Drawing for the job (mm, zero at the part's lowest x, y, z). Round coordinates to 2 decimals unless told otherwise and drop trailing zeros. Write each loop counter-clockwise with the first axis right and the second up, starting at its lowest first coordinate (ties: lowest second). Pieces come first, ordered by that corner, then holes.
Item 1: Drop flat-ended pins along their axis: pin 1 Ø15 at (y, z) = (586, 457) entering from -X; pin 2 Ø12 at (x, y) = (802, 277) entering from -Z. Give the stop position or say it passes through.
Item 2: Mould opens along X. For the marked faces 1 and 2 say: +X half, -X half, draft (parallel to the pull), parting line (faces both ways), or undercut.
Item 3: Wall check: probe 1 along X at (y, z) = (46.5, 217); probe 2 along Z at (x, y) = (641, 485). Give the ranges that are in metal, low to high.
Item 4: Band-saw the part on D-D, the plane x = 477.5. Write the cut outline in (y, z), then the cut area to 3 significant figures.
Item 5: Band-saw the part on B-B, the plane y = 532. Write the cut outline in (x, z).
Item 6: Band-saw the part on C-C, the plane y = 336. Write the cut outline in (x, z).
Item 7: Band-saw the part on A-A, the plane z = 806.5. Write the cut outline in (x, y).
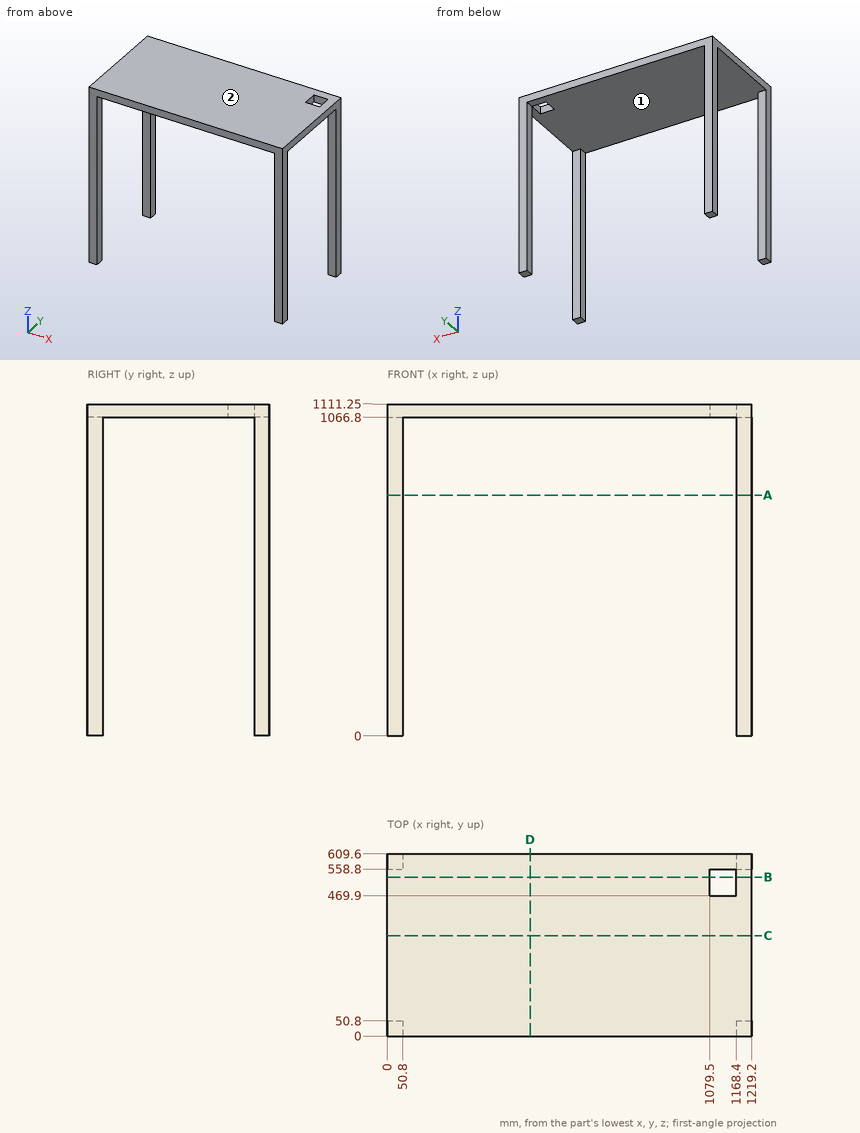
Results:
1. pin 1: stops at x = 0
1. pin 2: stops at z = 1066.8
2. face 1: undercut
2. face 2: draft
3. probe 1: x = 0 to 50.8, 1168.4 to 1219.2
3. probe 2: z = 1066.8 to 1111.25
4. outline: (0, 1066.8) - (609.6, 1066.8) - (609.6, 1111.25) - (0, 1111.25) - close
4. area: 27,100 mm2
5. outline: (0, 1066.8) - (1079.5, 1066.8) - (1079.5, 1111.25) - (0, 1111.25) - close; (1168.4, 1066.8) - (1219.2, 1066.8) - (1219.2, 1111.25) - (1168.4, 1111.25) - close
6. outline: (0, 1066.8) - (1219.2, 1066.8) - (1219.2, 1111.25) - (0, 1111.25) - close
7. outline: (0, 0) - (50.8, 0) - (50.8, 50.8) - (0, 50.8) - close; (0, 558.8) - (50.8, 558.8) - (50.8, 609.6) - (0, 609.6) - close; (1168.4, 0) - (1219.2, 0) - (1219.2, 50.8) - (1168.4, 50.8) - close; (1168.4, 558.8) - (1219.2, 558.8) - (1219.2, 609.6) - (1168.4, 609.6) - close
